Source: CAD feature listing. Evaluate the final solid. Frame: model axes, mm. A direction names the side the tool comes from. Coordinates: 2 decimals unless noted, no trailing zeros. Order: outer loops, then holes, each group sorted by start corner. A loop starts at its lowest first (then second) coordinate and runs counter-clockwise, first axis right, second up.
```python
from build123d import *

# Parameters (mm, degrees)
F0_R     = 2.25
F0_W     = 10
F0_H     = 10
F1_DEPTH = 3


# Not quite as in the source:
# - a feature names something its author has since deleted; it is built from what else it names


with BuildPart() as f1:
    # F0 (on Top) → F1 (new body)
    with BuildSketch(Plane.XY):
        Polygon((-50, -39.9732751399), (50, -39.9732751399), (50, 30.0267248601), (-40, 30.0267248601), (-50, 30.0267248601), align=None)
        with Locations((-40, -29.9732751399)):
            Circle(F0_R, mode=Mode.SUBTRACT)
        with Locations((40, -29.9732751399)):
            Circle(F0_R, mode=Mode.SUBTRACT)
        with BuildLine():
            Line((2.5, 4.1267248601), (2.5, 1.5650732754))
            ThreePointArc((2.5, 1.5650732754), (5.7662812973, -1.0046481733), (7, -4.9732751399))
            ThreePointArc((7, -4.9732751399), (-3.9686269666, -10.7395564373), (-2.5, 1.5650732754))
            Line((-2.5, 1.5650732754), (-2.5, 4.1267248601))
            Line((-2.5, 4.1267248601), (2.5, 4.1267248601))
        make_face(mode=Mode.SUBTRACT)
        with Locations((-40, 20.0267248601)):
            Circle(F0_R, mode=Mode.SUBTRACT)
        with Locations((40, 20.0267248601)):
            Circle(F0_R, mode=Mode.SUBTRACT)
        with Locations((-45, 35.0267248601)):
            Rectangle(F0_W, F0_H)
    extrude(amount=F1_DEPTH)


solid = f1.part
```
1. Section query A-A, the plane x = 40. Output: boundary loops of the cut face in (y, z).
2. Section query D-D, the plane y = 35. Output: boundary loops of the cut face in (x, z), plus the area to 3 significant figures.
3. Section query C-C, the plane z = 0.5. Output: boundary loops of the cut face in (x, y), plus the area to 3 significant figures.
4. Draft query along X for faces 4 (the flat face through (50, -5, 1)), 5 (the flat face through (-45, 40.027, 1)), 6 (the flat face through (-2.5, 3, 1)). Return one class per face: +X half, -X half, draft (parallel to the pull), parting line (faces both ways), or undercut.
5. Contact query for flat-ended pins moving along their axis: P1, Ø2.5, axis at x = -40, y = 20.03, coming from the +Z side; P2, Ø1.5, axis at y = 34, z = 2, coming from the +X side. Output: stop coordinate, or through.
6. Section query B-B, the plane x = 0. Output: boundary loops of the cut face in (y, z).
7. Material intervals for line 1 along Y through (x, z) = (40, 1.6); line 2 along X through (y, z) = (22, 0.55); line 3 along Y through (x, z) = (39.5, 1.95), sorted ascending.
8. Access query for faces 1 (the flat face through (-12, 1, 3)), 2 (the flat face through (0, 4.127, 1)), 3 (the flat face through (-40, 35, 1)). Directions: +Z, -Z, +X, -X, +Y, -Y. A direction counts if a zero-diameter tool reaches every point of the face in a straight line with its end or side. Return the directions, or none.
Answer key:
1. outline: (-39.97, 0) - (-32.22, 0) - (-32.22, 3) - (-39.97, 3) - close; (-27.72, 0) - (17.78, 0) - (17.78, 3) - (-27.72, 3) - close; (22.28, 0) - (30.03, 0) - (30.03, 3) - (22.28, 3) - close
2. outline: (-50, 0) - (-40, 0) - (-40, 3) - (-50, 3) - close
2. area: 30.0 mm2
3. outline: (-50, -39.97) - (50, -39.97) - (50, 30.03) - (-40, 30.03) - (-40, 40.03) - (-50, 40.03) - close; hole circle Ø4.5 at (-40, -29.97); hole circle Ø4.5 at (-40, 20.03); hole (-2.5, 1.57) arc R7 ccw (long way) to (2.5, 1.57) - (2.5, 4.13) - (-2.5, 4.13) - close; hole circle Ø4.5 at (40, -29.97); hole circle Ø4.5 at (40, 20.03)
3. area: 6,870 mm2
4. face 4: +X half
4. face 5: draft
4. face 6: undercut
5. P1: passes through
5. P2: stops at x = -40
6. outline: (-39.97, 0) - (-11.97, 0) - (-11.97, 3) - (-39.97, 3) - close; (4.13, 0) - (30.03, 0) - (30.03, 3) - (4.13, 3) - close
7. line 1: y = -39.97 to -32.22, -27.72 to 17.78, 22.28 to 30.03
7. line 2: x = -50 to -41.08, -38.92 to 38.92, 41.08 to 50
7. line 3: y = -39.97 to -32.17, -27.78 to 17.83, 22.22 to 30.03
8. face 1: +Z, +X, -X, +Y, -Y
8. face 2: +Z, -Z
8. face 3: +Z, -Z, +X, +Y
